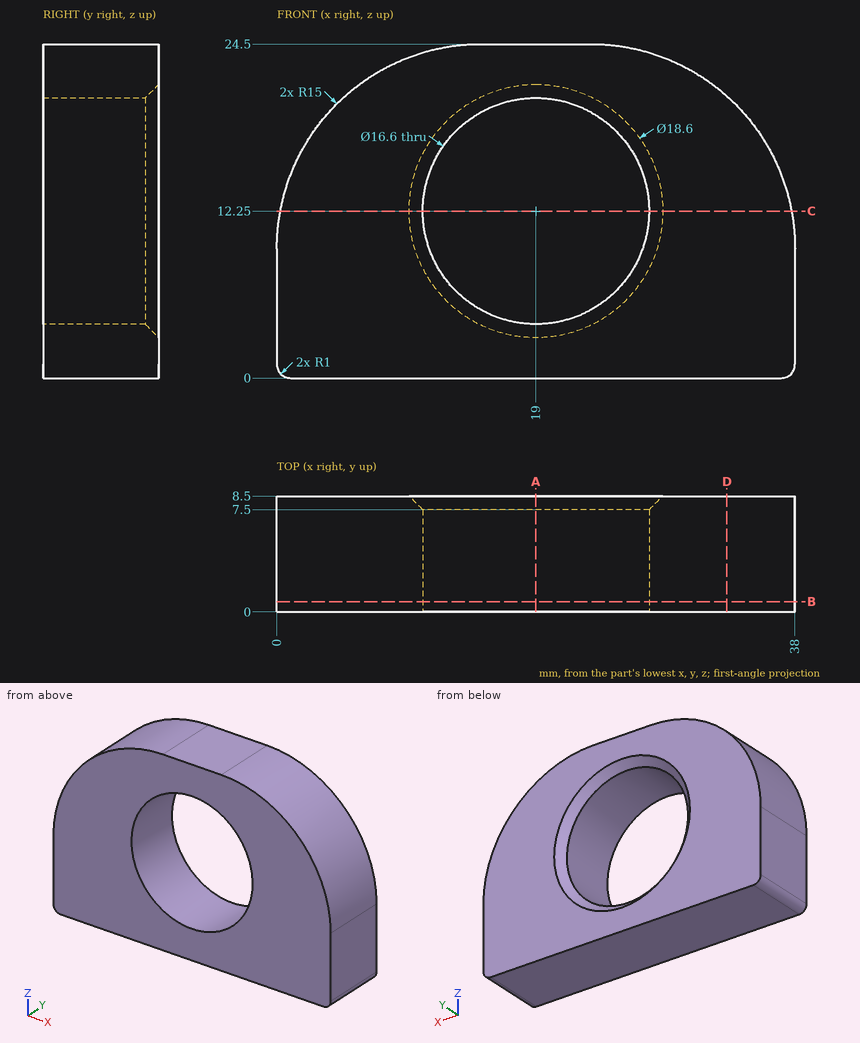
Answer from the drawing. Dimensions are ordinates in mm from the lowest x, y and z of the part. Coordinates: 2 decimals unless noted, no trailing zeros. Loops run counter-clockwise (first coordinate to the right, second up) from the corner with the lowest first, then second, coordinate; pieces in that order, holes last. Notation, with made-up numbers: (73.5, -19) -> (124.5, -19) arc R18 ccw to (124.5, -12) -> close; hole circle Ø11 at (33.5, 31). An arc over 180 degrees is marked (long way). Answer in a Markdown table with one row per item.
Item 1: A cutting plane is placed at C-C on z = 12.25. Determine the outline of the cut face in (x, y), plus the area to 3 significant figures.
Returned:
| item | result |
|---|---|
| outline | (0.25, 0) -> (10.7, 0) -> (10.7, 7.5) -> (9.7, 8.5) -> (0.25, 8.5) -> close; (27.3, 0) -> (37.75, 0) -> (37.75, 8.5) -> (28.3, 8.5) -> (27.3, 7.5) -> close |
| area | 177 mm^2 |
Item 2: A cutting plane is placed at A-A on x = 19. Determine the outline of the cut face in (y, z).
Returned:
| item | result |
|---|---|
| outline | (0, 0) -> (8.5, 0) -> (8.5, 2.95) -> (7.5, 3.95) -> (0, 3.95) -> close; (0, 20.55) -> (7.5, 20.55) -> (8.5, 21.55) -> (8.5, 24.5) -> (0, 24.5) -> close |
Item 3: Straight lines are drawn through the part: line 1 along X through (y, z) = (3.5, 12.25); line 2 along X through (y, z) = (1.75, 8.75); line 3 along Z through (x, y) = (16, 8). For each, find the intervals that lie inside material, in ascending order. Write a range as [from, to].
Returned:
| item | result |
|---|---|
| line 1 | x = [0.25, 10.7], [27.3, 37.75] |
| line 2 | x = [0, 11.47], [26.53, 38] |
| line 3 | z = [0, 3.98], [20.52, 24.5] |
Item 4: A cutting plane is placed at D-D on x = 33. Determine the outline of the cut face in (y, z).
Returned:
| item | result |
|---|---|
| outline | (0, 0) -> (8.5, 0) -> (8.5, 20.68) -> (0, 20.68) -> close |
Item 5: A cutting plane is placed at B-B on y = 0.75. Determine the outline of the cut face in (x, z), plus the area to 3 significant figures.
Returned:
| item | result |
|---|---|
| outline | (0, 1) arc R1 ccw to (1, 0) -> (37, 0) arc R1 ccw to (38, 1) -> (38, 9.5) arc R15 ccw to (23, 24.5) -> (15, 24.5) arc R15 ccw to (0, 9.5) -> close; hole circle Ø16.6 at (19, 12.25) |
| area | 618 mm^2 |
Item 6: This flat-tipped pin is pushed along its axis until it touches: P1, Ø1.5, axis at y = 2, z = 21.5, coming from the +X side. Where does it stop, or does it pass through?
Returned:
| item | result |
|---|---|
| P1 | stops at x = 32.92 |
